```python
from build123d import *

# Parameters (mm, degrees)
F0_W     = 12
F0_H     = 25
F0_W_2   = 7
F0_H_2   = 14
F0_R     = 2
F1_DEPTH = 20
F2_R     = 1
F3_DEPTH = 12.001


with BuildPart() as f1:
    # F0 (on Top) → F1 (new body)
    with BuildSketch(Plane.XY):
        with Locations((0, -7.5)):
            Rectangle(F0_W, F0_H)
        with Locations((0, -10)):
            Rectangle(F0_W_2, F0_H_2, mode=Mode.SUBTRACT)
        Circle(F0_R, mode=Mode.SUBTRACT)
    extrude(amount=F1_DEPTH)

    # F2 (on face) → F3 (cut, through all)
    with BuildSketch(Plane(origin=(-6, 0, 0), x_dir=(0, -1, 0), z_dir=(-1, 0, 0))):
        with Locations((13.5, 15)):
            Circle(F2_R)
        with Locations((6.5, 15)):
            Circle(F2_R)
        with Locations((7.5, 5)):
            Circle(F2_R)
    extrude(amount=-F3_DEPTH, mode=Mode.SUBTRACT)


solid = f1.part
```
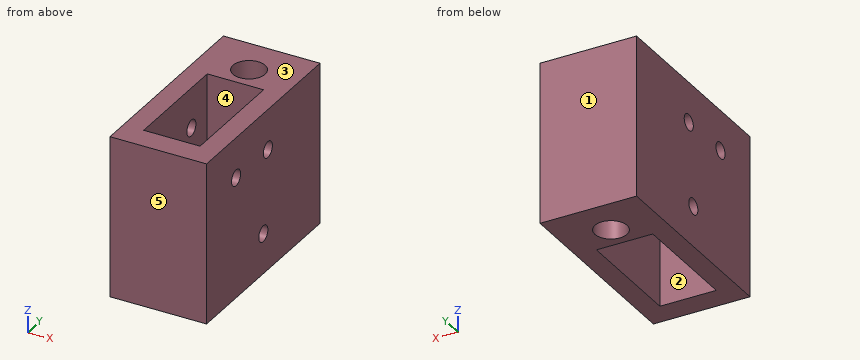
Geometry check sheet. Reference: the model listing, model coordinates, mm. Face numbers are marked on the shaded views. A direction names the side the tool comes from. Coordinates: 2 decimals unless noted, no trailing zeros. Loops run counter-clockwise (first coordinate to the right, second up) from the corner with the lowest first, then second, coordinate; pieces in that order, holes last.
Item 1: Thickness scan on line 1 (X direction, y = -8.75, z = 5.25); line 2 (Y direction, x = 0, z = 4.25); line 3 (Y direction, x = 1.5, z = 6.5). Record the ranges inside material, lowest first.
Item 2: Release check for a two-part mould opening along Y. For the marked faces 1, 2 and 3 record: released by +Y, released by -Y, zero draft, split by the parting line, or undercut.
Item 3: Sectioned sample at D-D, the plane y = 0. Record the boundary of the cut face in (x, z), then the cut area to 3 significant figures.
Item 4: Go/stop test with a flat-tipped pin: pin 1 Ø1.6 at (y, z) = (-6.5, 15) entering from +X. Record where the tip stops, or that it passes through.
Item 5: Sectioned sample at C-C, the plane z = 5. Record the boundary of the cut face in (x, y), then the cut area to 3 significant figures.
Item 6: Access from +Z, -Z, +X, -X, +Y, -Y to the whole of each face (thin tool, end or side, straight path). Record for the marked faces 4 and 5.
Item 7: Sectioned sample at A-A, the plane z = 15. Record the boundary of the cut face in (x, y), then the cut area to 3 significant figures.
Item 8: Sectioned sample at B-B, the plane x = 2.5. Record the boundary of the cut face in (y, z).
Check result:
1. line 1: x = -6 to -3.5, 3.5 to 6
1. line 2: y = -20 to -17, -3 to -2, 2 to 5
1. line 3: y = -20 to -17, -3 to -1.32, 1.32 to 5
2. face 1: released by +Y
2. face 2: undercut
2. face 3: zero draft
3. outline: (-6, 0) - (-2, 0) - (-2, 20) - (-6, 20) - close; (2, 0) - (6, 0) - (6, 20) - (2, 20) - close
3. area: 160 mm2
4. pin 1: passes through
5. outline: (-6, -20) - (6, -20) - (6, -8.5) - (3.5, -8.5) - (3.5, -17) - (-3.5, -17) - (-3.5, -8.5) - (-6, -8.5) - close; (-6, -6.5) - (-3.5, -6.5) - (-3.5, -3) - (3.5, -3) - (3.5, -6.5) - (6, -6.5) - (6, 5) - (-6, 5) - close; hole circle Ø4 at (0, 0)
5. area: 179 mm2
6. face 4: +Z, -Z
6. face 5: +Z, -Z, +X, -X, -Y
7. outline: (-6, -20) - (6, -20) - (6, -14.5) - (3.5, -14.5) - (3.5, -17) - (-3.5, -17) - (-3.5, -14.5) - (-6, -14.5) - close; (-6, -12.5) - (-3.5, -12.5) - (-3.5, -7.5) - (-6, -7.5) - close; (-6, -5.5) - (-3.5, -5.5) - (-3.5, -3) - (3.5, -3) - (3.5, -5.5) - (6, -5.5) - (6, 5) - (-6, 5) - close; (3.5, -12.5) - (6, -12.5) - (6, -7.5) - (3.5, -7.5) - close; hole circle Ø4 at (0, 0)
7. area: 169 mm2
8. outline: (-20, 0) - (-17, 0) - (-17, 20) - (-20, 20) - close; (-3, 0) - (5, 0) - (5, 20) - (-3, 20) - close
